```python
from build123d import *

# Parameters (mm, degrees)
SM_BASE_FLANGE_1_DEPTH = 1
CUT_EXTRUDE_1_DEPTH    = 10
CUT_EXTRUDE_2_DEPTH    = 10


# Sheet-metal steps are written as plain solids
with BuildPart() as part:
    # Sketch 1 → Базовая кромка1 (new body)
    with BuildSketch(Plane(origin=(0, 0, 0), x_dir=(1, 0, 0), z_dir=(0, 1, 0))):
        Polygon((-58.513846144, -161.889640506), (-212.364567845, -161.889640506), (-220.864567845, -153.389640506), (-222.278781408, -153.389640506), (-264.356991895, -153.389640506), (-295.11077987, -184.143428482), (-295.11077987, -227.635852531), (-264.356991895, -258.389640506), (-222.278781408, -258.389640506), (-220.864567845, -258.389640506), (-212.364567845, -249.889640506), (-58.513846144, -249.889640506), (-46.013846144, -262.389640506), (-44.599632582, -262.389640506), (0.278072842, -262.389640506), (33.88922013, -228.778493218), (33.88922013, -182.800787794), (0.478072842, -149.389640506), (-44.599632582, -149.389640506), (-46.013846144, -149.389640506), align=None)
    extrude(amount=-SM_BASE_FLANGE_1_DEPTH)

    # Эскиз3 → Вырез-Вытянуть1 (cut)
    with BuildSketch(Plane(origin=(0, 0, 0), x_dir=(1, 0, 0), z_dir=(0, 1, 0))):
        Polygon((-129.650630124, -194.854768426), (-112.66234875, -177.866487052), (-6.632911498, -177.866487052), (10.895241956, -195.394640506), (10.895241956, -217.265248922), (-6.633389706, -233.712753004), (-112.662389706, -233.712753004), (-129.650630124, -216.724512586), align=None)
    extrude(amount=-CUT_EXTRUDE_1_DEPTH, mode=Mode.SUBTRACT)

    # Эскиз4 → Вырез-Вытянуть2 (cut)
    with BuildSketch(Plane(origin=(0, 0, 0), x_dir=(1, 0, 0), z_dir=(0, 1, 0))):
        Polygon((-264.253438504, -153.639640506), (-216.125737308, -153.639640506), (-216.125737308, -129.066031108), (-310.48708542, -129.066031108), (-310.48708542, -280.318410607), (-216.781479831, -280.318410607), (-216.781479831, -258.139640506), (-264.253438504, -258.139640506), (-294.86077987, -227.53229914), (-294.86077987, -184.246981872), align=None)
        Polygon((-47.513022755, -149.639640506), (0.374519451, -149.639640506), (33.63922013, -182.904341185), (33.63922013, -228.674939827), (0.174519451, -262.139640506), (-50.1499885, -262.139640506), (-50.1499885, -286.805350845), (64.547971273, -286.805350845), (64.547971273, -129.066031108), (-47.513022755, -129.066031108), align=None)
    extrude(amount=-CUT_EXTRUDE_2_DEPTH, mode=Mode.SUBTRACT)


solid = part.part
```
The listing builds one solid part. Answer for the finished solid, in the listing's coordinates (mm). A direction names the side the tool comes from. Coordinates: 2 decimals unless noted, no trailing zeros. Loops run counter-clockwise (first coordinate to the right, second up) from the corner with the lowest first, then second, coordinate; pieces in that order, holes last. Notation, with made-up numbers: (19.25, -15.75) - (30.25, -15.75) arc R32 ccw to (30.25, 16.25) - close; hole circle Ø2 at (-26.75, -34). An arc over 180 degrees is marked (long way). Use a Markdown table: item, result. Add a question column.
1) The part is cut by section D-D, the plane x = -195.5. Give the vertices of the cut face in (y, z).
2) The part is cut by section A-A, the plane z = 210. Give the vertices of the cut face in (x, y).
3) The part is cut by section B-B, the plane x = -77.5. Give the vertices of the cut face in (y, z), and give its area (3 significant figures).
4) Find the intervals of material crossed by line 1 (Z direction, x = -11.5, y = -0.7); line 2 (X direction, y = -0.4, z = 213); line 3 (Z direction, x = -86, y = -0.4), in increasing order.
5) The part is cut by section C-C, the plane y = -0.6. Give the vertices of the cut face in (x, z), and give its area (3 significant figures).
6) For faces 5 (the flat face through (-52.475, -0.493, 255.929)), 6 (the flat face through (-121.038, -0.493, 225.338)), 7 (the flat face through (-52.303, -0.493, 155.679)), determine the directions among +Z, -Z, +X, -X, +Y, -Y from which every point of the face is accessible in a straight line to the end or side of a thin tool.
7) The mould has two halves that part along Z. Classify faces 1 (the flat face through (-169, 0, 205)), 2 (the flat face through (-216.432, -0.493, 157.822)), 3 (the flat face through (2.254, -0.493, 225.374)), 4 (the flat face through (17.141, -0.493, 245.173)): released by +Z, released by -Z, zero draft, split by the parting line, or undercut.
Here are the results:
| question | item | result |
|---|---|---|
| 1 | outline | (-1, 161.89) - (0, 161.89) - (0, 249.89) - (-1, 249.89) - close |
| 2 | outline | (-294.86, -1) - (-129.65, -1) - (-129.65, 0) - (-294.86, 0) - close; (10.9, -1) - (33.64, -1) - (33.64, 0) - (10.9, 0) - close |
| 3 | outline | (-1, 161.89) - (0, 161.89) - (0, 177.87) - (-1, 177.87) - close; (-1, 233.71) - (0, 233.71) - (0, 249.89) - (-1, 249.89) - close |
| 3 | area | 32.2 mm^2 |
| 4 | line 1 | z = 149.64 to 177.87, 233.71 to 262.14 |
| 4 | line 2 | x = -294.86 to -129.65, 10.9 to 33.64 |
| 4 | line 3 | z = 161.89 to 177.87, 233.71 to 249.89 |
| 5 | outline | (-294.86, 184.25) - (-264.25, 153.64) - (-220.61, 153.64) - (-212.36, 161.89) - (-58.51, 161.89) - (-46.26, 149.64) - (0.37, 149.64) - (33.64, 182.9) - (33.64, 228.67) - (0.17, 262.14) - (-46.26, 262.14) - (-58.51, 249.89) - (-212.36, 249.89) - (-220.61, 258.14) - (-264.25, 258.14) - (-294.86, 227.53) - close; hole (-129.65, 194.85) - (-112.66, 177.87) - (-6.63, 177.87) - (10.9, 195.39) - (10.9, 217.27) - (-6.63, 233.71) - (-112.66, 233.71) - (-129.65, 216.72) - close |
| 5 | area | 23,000 mm^2 |
| 6 | face 5 | +Z, +Y, -Y |
| 6 | face 6 | +Y, -Y |
| 6 | face 7 | -Z, +Y, -Y |
| 7 | face 1 | zero draft |
| 7 | face 2 | released by -Z |
| 7 | face 3 | undercut |
| 7 | face 4 | released by +Z |
